Build history of the part. All positions in model axes, mm. A direction names the side the tool comes from. Round coordinates to 2 decimals unless told otherwise and drop trailing zeros. Write each loop counter-clockwise with the first axis right and the second up, starting at its lowest first coordinate (ties: lowest second). Pieces come first, ordered by that corner, then holes. Notation, with made-up numbers: M 1,62.5 L 13,62.5 A20 ccw 13,99.5 Z; hole C -38.75,42.5 d4. An arc over 180 degrees is marked long. One line per item, written item: value. Start each with the question number.
Solid Edge part; units mm, degrees
sketch "Sketch1" plane through (0, 0, 0) normal (1, 0, 0) x (0, 1, 0)
  line L0 (11.7, -6.65) -> (16.85, -6.65)
  line L1 (16.85, -6.65) -> (16.85, -5.0543)
  line L2 (16.85, -5.0543) -> (35.15, -5.0543)
  line L3 (35.15, -5.0543) -> (35.15, -6.65)
  line L4 (35.15, -6.65) -> (40.3503, -6.65)
  line L5 (40.3503, -6.65) -> (40.3503, -10)
  line L6 (40.3503, -10) -> (11.7, -10)
  line L7 (11.7, -10) -> (11.7, -6.65)
revolve "RevolvedProtrusion1" add sketch "Sketch1" angle 360 about axis through (0, -60, 0) along (0, 1, 0)
sketch "Sketch2" plane through (0, 0, 0) normal (1, 0, 0) x (0, 1, 0)
  line L0 (11.7, -10) -> (40.3503, -10)
  line L1 (40.3503, 0) -> (40.3503, -10)
  line L2 (11.7, 0) -> (40.3503, 0)
  line L3 (11.7, 0) -> (11.7, -10)
extrude "Protrusion1" add sketch "Sketch2" along normal mid plane 20
sketch "Sketch3" plane through (0, 0, 0) normal (1, 0, 0) x (0, 1, 0)
  line L0 (11.7, 0) -> (11.7, 6.65)
  line L1 (11.7, 6.65) -> (16.85, 6.65)
  line L2 (16.85, 5.0543) -> (16.85, 6.65)
  line L3 (16.85, 5.0543) -> (35.15, 5.0543)
  line L4 (35.15, 5.0543) -> (35.15, 6.65)
  line L5 (35.15, 6.65) -> (40.3503, 6.65)
  line L6 (40.3503, 0) -> (40.3503, 6.65)
  line L7 (11.7, 0) -> (40.3503, 0)
revolve "RevolvedCutout_1" cut sketch "Sketch3" angle 284.342 about axis through (0, -60, 0) along (0, 1, 0)
sketch "Sketch4" plane through (0, 11.7, 0) normal (0, -1, 0) x (1, 0, 0)
  line L0 (-12.0207, 0) -> (12.5476, 0)
  line L1 (12.5476, 0) -> (12.5476, 10.6039)
  line L2 (12.5476, 10.6039) -> (-12.0207, 10.6039)
  line L3 (-12.0207, 10.6039) -> (-12.0207, 0)
extrude "ExtrudedCutout_1" cut sketch "Sketch4" against normal blind 426.8623
sketch "Sketch5" plane through (-10, 26.0252, -5) normal (-1, 0, 0) x (0, -1, 0)
  line L0 (-15.9005, 5) -> (15.9429, 5)
  line L1 (15.9429, 5) -> (15.9429, 4)
  line L2 (15.9429, 4) -> (-15.9005, 4)
  line L3 (-15.9005, 4) -> (-15.9005, 5)
extrude "ExtrudedCutout_2" cut sketch "Sketch5" against normal blind 53.8114
sketch "Sketch6" plane through (-7.4772, 26.0252, -1) normal (0, 0, 1) x (0, -1, 0)
  line L0 (-14.3252, -2.5228) -> (14.3252, -2.5228)
  line L1 (14.3252, -2.5228) -> (14.3252, -9.4972)
  line L2 (14.3252, -9.4972) -> (-14.3252, -9.4972)
  line L3 (-14.3252, -9.4972) -> (-14.3252, -2.5228)
  dimension "D1" = 14.3252
extrude "Protrusion2" add sketch "Sketch6" against normal up to vertex (9 mm away)
mirror "Mirror1" about plane through (0, 0, 0) normal (1, 0, 0) of "Protrusion2"
sketch "Sketch7" plane through (-10.9644, 26.0252, -1) normal (0, 0, 1) x (1, 0, 0)
  circle A0 centre (-0.81, -9.1252) radius 2.2
  circle A1 centre (22.7388, -9.1252) radius 2.2
  circle A2 centre (-0.81, 9.1252) radius 2.2
  circle A3 centre (22.7388, 9.1252) radius 2.2
extrude "ExtrudedCutout_3" cut sketch "Sketch7" against normal blind 291.9173
Item 1: Two-plate mould, pull along Y, no slides. Class faces 1 (the cylindrical face through (11.3, 14.75, -5.44)), 2 (the flat face through (-11, 26, -1)), 3 (the cylindrical face through (11.297, 33.003, -5.437)), 4 (the flat face through (-14, 40.35, -5)): pulls with the +Y half, pulls with the -Y half, needs draft (parallel to the pull), parting line crosses it, or undercut.
Item 2: Cut at A-A, the plane z = -1.5. Count the separate pieces of the cut face and the enclosed holes in it, plus the area to 3 significant figures.
Item 3: Cut at B-B, the plane x = 13. Write the cut outline in (y, z).
Item 4: Drop flat-ended pins along their axis: pin 1 (4 mm diameter, centred on x = 11.77, y = 35.15, fed in from +Z); pin 2 (2 mm diameter, centred on x = 2.5, z = -4.5, fed in from +Y); pin 3 (3 mm diameter, centred on x = -2, z = -3.5, fed in from -Y). Give the stop position or say it passes through.
Item 5: Which spindle directions (+Z, -Z, +X, -X, +Y, -Y) get a long thin tool onto all of the face, cutting with end or side? Do faces 5 (the cylindrical face through (-12.251, 33.003, -5.437)), 6 (the cylindrical face through (0.13, 14.31, -6.65)), 7 (the flat face through (0.5, 35.15, -5.3)). Say none if no direction does.
Item 6: Cut at C-C, the plane y = 18. Write the cut outline in (x, z).
Item 7: Drill centre lines: line 1 (Y direction, x = -11.5, z = -9.5); line 2 (X direction, y = 17.25, z = -8.75); line 3 (X direction, y = 36.25, z = -5.5). Where is each one in solid material? Low to high.
Computed values:
1. face 1: undercut
1. face 2: needs draft
1. face 3: undercut
1. face 4: pulls with the +Y half
2. separate pieces: 2
2. enclosed holes: 4
2. area: 601 mm2
3. outline: M 11.7,-10 L 15.07,-10 L 15.07,-1 L 11.7,-1 Z; M 18.73,-10 L 33.32,-10 L 33.32,-1 L 18.73,-1 Z; M 36.98,-10 L 40.35,-10 L 40.35,-1 L 36.98,-1 Z
4. pin 1: passes through
4. pin 2: stops at y = 35.15
4. pin 3: stops at y = 16.85
5. face 5: +Z, -Z
5. face 6: +Z, -Y
5. face 7: +Z, +Y
6. outline: M -16.97,-10 L -13.68,-10 L -13.68,-1 L -16.97,-1 Z; M -9.87,-10 L 9.87,-10 L 9.87,-1 L 4.95,-1 A5.05 cw -4.95,-1 L -9.87,-1 Z; M 13.68,-10 L 16.97,-10 L 16.97,-1 L 13.68,-1 Z
7. line 1: y = 11.7 to 14.72, 19.08 to 32.97, 37.33 to 40.35
7. line 2: x = -16.97 to -13.95, -9.6 to 9.6, 13.95 to 16.97
7. line 3: x = -16.97 to -13.68, -9.87 to -3.74, 3.74 to 9.87, 13.68 to 16.97
